Design review of the part built by this model. Coordinates are the model's own, in mm. A direction names the side the tool comes from. Coordinates: 2 decimals unless noted, no trailing zeros. Order: outer loops, then holes, each group sorted by start corner. A loop starts at its lowest first (then second) coordinate and runs counter-clockwise, first axis right, second up. Notation, with made-up numbers: M 38,-28.75 L 80,-28.75 A3 cw 80,-23.75 Z; hole C 16,24 d7. An arc over 180 degrees is marked long. Answer in a Markdown table with one row per item.
from build123d import *

# Parameters (mm, degrees)
SKETCH1_W           = 38
SKETCH1_H           = 24.5
SKETCH1_R           = 8.075
BOSS_EXTRUDE1_DEPTH = 3
FILLET1_R           = 15
SKETCH3_W           = 1.4
SKETCH3_H           = 1.4
FILLET2_R           = 1
CHAMFER1_SIZE       = 0.5


with BuildPart() as part:
    # Sketch1 → Boss-Extrude1 (new body)
    with BuildSketch(Plane(origin=(0, 0, 0), x_dir=(1, 0, 0), z_dir=(0, 1, 0))):
        Rectangle(SKETCH1_W, SKETCH1_H)
        with Locations(Location((0, 0, 0), (0, 0, 270))):
            Circle(SKETCH1_R, mode=Mode.SUBTRACT)
    extrude(amount=BOSS_EXTRUDE1_DEPTH)

    # Fillet1
    fillet1_edges = [part.edges().sort_by_distance(p)[0] for p in [
        (19, 1.5, 12.25),
        (-19, 1.5, 12.25),
    ]]
    fillet(fillet1_edges, radius=FILLET1_R)

    # Cut-Sweep1: sweep along a path in Sketch2
    with BuildLine(Plane(origin=(0, 3, 0), x_dir=(1, 0, 0), z_dir=(0, 1, 0))) as cut_sweep1_path:
        CenterArc((0, 0), 10.5, 0, 360)
    # Sketch3 → Cut-Sweep1 (sweep, cut)
    with BuildSketch(Plane.XY):
        with Locations((10.5, 3)):
            Rectangle(SKETCH3_W, SKETCH3_H)
    sweep(path=cut_sweep1_path.line, mode=Mode.SUBTRACT)

    # Fillet2
    fillet2_edges = [part.edges().sort_by_distance(p)[0] for p in [
        (-19, 1.5, -12.25),
        (19, 1.5, -12.25),
    ]]
    fillet(fillet2_edges, radius=FILLET2_R)

    # Chamfer1
    chamfer1_edges = [part.edges().sort_by_distance(p)[0] for p in [
        (0, 3, -8.075),
    ]]
    chamfer(chamfer1_edges, length=CHAMFER1_SIZE)


solid = part.part
(1) Draft analysis for pull direction Z (two halves, no side actions). For faces 1 (the flat face through (0, 1, -12.25)), 2 (the cylindrical face through (-14.72, 1.52, 7.74)), 3 (the flat face through (-0.3, 0, -8.3)), 4 (the cylindrical face through (-11.19, 2.65, -0.49)), state which applies: pulls with the +Z half, pulls with the -Z half, needs draft (parallel to the pull), parting line crosses it, or undercut.
Return value:
| item | result |
|---|---|
| face 1 | pulls with the -Z half |
| face 2 | pulls with the +Z half |
| face 3 | needs draft |
| face 4 | undercut |
(2) For line 1 along Z through (x, y) = (-5, 2.75); line 2 along X through (y, z) = (2.8, 0) (3 decimals); line 3 along X through (y, z) = (2.4, -7.25), list the stretches that pass through material, from the lowest coordinate up. Write a range as from..to.
Return value:
| item | result |
|---|---|
| line 1 | z = -12.25..-10.02, -8.43..-6.66, 6.66..8.43, 10.02..12.22 |
| line 2 | x = -18.746..-11.2, -9.8..-8.375, 8.375..9.8, 11.2..18.746 |
| line 3 | x = -19..-8.54, -6.59..-3.56, 3.56..6.59, 8.54..19 |
(3) For faces 5 (the flat face through (0, 1, 12.25)), 6 (the cylindrical face through (-2.124, 2.645, 9.567)), list the 3-axis set-ups (+Z, -Z, +X, -X, +Y, -Y) from which the entire face can be reached by the end or side of a thin tool; tool diameter is ignored.
Return value:
| item | result |
|---|---|
| face 5 | +Z, +X, -X, +Y, -Y |
| face 6 | +Y |
(4) Add section B-B, the plane x = 13.5. Give the boundary of the cut face in (y, z), and give its area (3 significant figures).
Return value:
| item | result |
|---|---|
| outline | M 0,-12.25 L 3,-12.25 L 3,8.86 L 0,8.86 Z |
| area | 63.3 mm2 |
(5) Add section A-A, the plane y = 0.95. Give the boundary of the cut face in (x, z) (3 decimals).
Return value:
| item | result |
|---|---|
| outline | M -19,-11.25 A1 ccw -18,-12.25 L 18,-12.25 A1 ccw 19,-11.25 L 19,-2.75 A15 ccw 4,12.25 L -4,12.25 A15 ccw -19,-2.75 Z; hole C 0,0 d16.15 |
